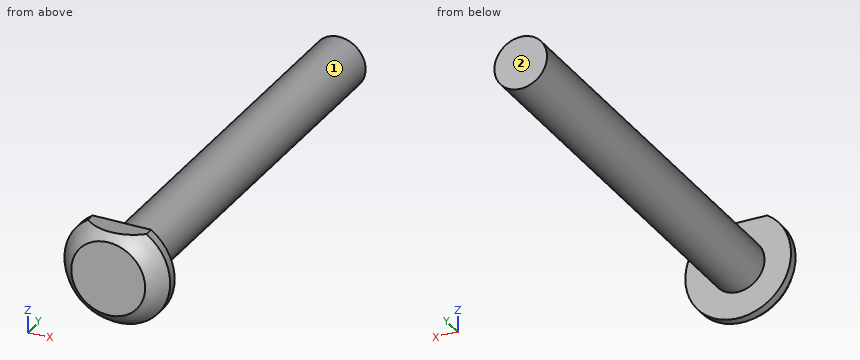
```python
from build123d import *

# Parameters (mm, degrees)
F3_DEPTH = 4.7625


with BuildPart() as f1:
    # F0 (on Right) → F1 (revolve)
    with BuildSketch(Plane.YZ):
        with BuildLine():
            Line((-1.5875, 0), (0, 0))
            Line((0, 0), (76.2, 0))
            Line((76.2, 0), (76.2, 4.74345))
            Line((76.2, 4.74345), (0, 4.74345))
            Line((0, 4.74345), (0, 9.525))
            Line((0, 9.525), (-1.5875, 9.525))
            ThreePointArc((-1.5875, 9.525), (-3.314423, 8.244646), (-4.7625, 6.655734))
            Line((-4.7625, 6.655734), (-4.7625, 0))
            Line((-4.7625, 0), (-1.5875, 0))
        make_face()
    revolve(axis=Axis((0, 38.1, 0), (0, 1, 0)))

    # F2 (on face) → F3 (cut)
    with BuildSketch(Plane.XZ.offset(4.7625)):
        with BuildLine():
            ThreePointArc((5.299691, 7.9375), (0, 9.544141), (-5.299691, 7.9375))
            Line((-5.299691, 7.9375), (5.299691, 7.9375))
        make_face()
    extrude(amount=-F3_DEPTH, mode=Mode.SUBTRACT)


solid = f1.part
```
Geometry: final body of the model. Coordinates: model frame, mm. Face numbers are marked on the shaded views. A direction names the side the tool comes from. Coordinates: 2 decimals unless noted, no trailing zeros. Order: outer loops, then holes, each group sorted by start corner. A loop starts at its lowest first (then second) coordinate and runs counter-clockwise, first axis right, second up. Notation, with made-up numbers: (86, 22.5) - (98, 22.5) arc R16 cw to (98, 38.5) - close; hole circle Ø2 at (40.25, 16). An arc over 180 degrees is marked (long way). Write each question's results on one line, items separated by ' | '.
1) Set-up query: the marked faces 1 and 2. Return all of +Z, -Z, +X, -X, +Y, -Y with unobstructed straight access to the full face (end or side cutting, diameter ignored); none if empty.
Results list:
face 1: +Y | face 2: +Z, -Z, +X, -X, +Y
2) Line query: line 1 (Z direction, x = 0.25, y = 53.5); line 2 (Y direction, x = 0, z = 6.75); line 3 (X direction, y = 69, z = 3.5). Output: solid intervals per line, ascending. Write a range as from..to.
Results list:
line 1: -4.74..4.74 | line 2: -4.69..0 | line 3: -3.2..3.2
3) Section A-A, the plane y = 38. Return loops of the section in (x, z).
Results list:
outline: circle Ø9.49 at (0, 0)
4) Pin query (flat end, axial travel): pin 1 (4 mm diameter, centred on y = 18, z = 4.5, fed in from -X); pin 2 (3 mm diameter, centred on x = -4.5, y = 54.5, fed in from -Z); pin 3 (1 mm diameter, centred on x = -6, y = 56, fed in from +Z); pin 4 (3 mm diameter, centred on x = 2, y = 37, fed in from +Z). Return the tip coordinate at first contact, or that it passes through.
Results list:
pin 1: x = -4.03 | pin 2: z = -3.67 | pin 3: through | pin 4: z = 4.72
